from build123d import *

# Parameters (mm, degrees)
SKETCH1_W                  = 330
SKETCH1_H                  = 40
BOSS_EXTRUDE1_DEPTH        = 10
SKETCH2_W                  = 10.95
SKETCH2_H                  = 9
SKETCH2_W_2                = 8.1
SKETCH2_H_2                = 6.6
SKETCH2_H_3                = 6.8
SKETCH2_W_3                = 2.5
SKETCH2_H_4                = 4.6
CUT_EXTRUDE1_DEPTH         = 167.508258053
FILLET1_R                  = 2.5
LPATTERN1_COUNT            = 3
LPATTERN1_PITCH            = 70
FILLET1_OF_LPATTERN1_R     = 2.5
LPATTERN1_COL_COUNT        = 3
LPATTERN1_COL_PITCH        = 70
FILLET1_OF_LPATTERN1_COL_R = 2.5
SKETCH3_W                  = 10
SKETCH3_H                  = 9
CUT_EXTRUDE2_DEPTH         = 167.508258053
FILLET2_R                  = 20


with BuildPart() as part:
    # Sketch1 → Boss-Extrude1 (new body)
    with BuildSketch(Plane(origin=(0, 0, 0), x_dir=(1, 0, 0), z_dir=(0, 1, 0))):
        Rectangle(SKETCH1_W, SKETCH1_H)
    extrude(amount=BOSS_EXTRUDE1_DEPTH)

    # Sketch2 → Cut-Extrude1 (cut, through all)
    with BuildSketch(Plane(origin=(0, 10, 0), x_dir=(1, 0, 0), z_dir=(0, 1, 0))):
        with Locations((9.525, -15.5)):
            Rectangle(SKETCH2_W, SKETCH2_H)
        with Locations((0, -15.5)):
            Rectangle(SKETCH2_W_2, SKETCH2_H)
        with Locations((-9.525, -15.5)):
            Rectangle(SKETCH2_W, SKETCH2_H)
        with Locations((0, -7.7)):
            Rectangle(SKETCH2_W_2, SKETCH2_H_2)
        with Locations((0, -1)):
            Rectangle(SKETCH2_W_2, SKETCH2_H_3)
        with Locations((-5.3, -1)):
            Rectangle(SKETCH2_W_3, SKETCH2_H_3)
        with Locations((0, 4.7)):
            Rectangle(SKETCH2_W_2, SKETCH2_H_4)
        with Locations((5.3, -1)):
            Rectangle(SKETCH2_W_3, SKETCH2_H_3)
    cut_extrude1 = extrude(amount=-CUT_EXTRUDE1_DEPTH, mode=Mode.SUBTRACT)

    # Fillet1
    fillet1_edges = [part.edges().sort_by_distance(p)[0] for p in [
        (15, 5, 20),
        (-15, 5, 20),
    ]]
    fillet(fillet1_edges, radius=FILLET1_R)

    # LPattern1: Cut-Extrude1 ×3
    with Locations(*[(i * LPATTERN1_PITCH, 0, 0) for i in range(1, LPATTERN1_COUNT)]):
        add(cut_extrude1, mode=Mode.SUBTRACT)

    # Fillet1 of LPattern1
    fillet1_of_lpattern1_edges = [part.edges().sort_by_distance(p)[0] for p in [
        (85, 5, 20),
        (55, 5, 20),
        (155, 5, 20),
        (125, 5, 20),
    ]]
    fillet(fillet1_of_lpattern1_edges, radius=FILLET1_OF_LPATTERN1_R)

    # LPattern1 col: Cut-Extrude1 ×3
    with Locations(*[(-i * LPATTERN1_COL_PITCH, 0, 0) for i in range(1, LPATTERN1_COL_COUNT)]):
        add(cut_extrude1, mode=Mode.SUBTRACT)

    # Fillet1 of LPattern1 col
    fillet1_of_lpattern1_col_edges = [part.edges().sort_by_distance(p)[0] for p in [
        (-55, 5, 20),
        (-85, 5, 20),
        (-125, 5, 20),
        (-155, 5, 20),
    ]]
    fillet(fillet1_of_lpattern1_col_edges, radius=FILLET1_OF_LPATTERN1_COL_R)

    # Sketch3 → Cut-Extrude2 (cut, through all)
    with BuildSketch(Plane(origin=(0, 10, 0), x_dir=(1, 0, 0), z_dir=(0, 1, 0))):
        with Locations((-160, -15.5)):
            Rectangle(SKETCH3_W, SKETCH3_H)
    cut_extrude2 = extrude(amount=-CUT_EXTRUDE2_DEPTH, mode=Mode.SUBTRACT)

    # Mirror1: Cut-Extrude2 across plane
    add(cut_extrude2.mirror(Plane(origin=(0, 0, 0), x_dir=(0, 0, 1), z_dir=(1, 0, 0))), mode=Mode.SUBTRACT)

    # Fillet2
    fillet2_edges = [part.edges().sort_by_distance(p)[0] for p in [
        (-165, 5, -20),
        (165, 5, -20),
    ]]
    fillet(fillet2_edges, radius=FILLET2_R)


solid = part.part
Design review of the part built by this model. Coordinates are the model's own, in mm. A direction names the side the tool comes from. Coordinates: 2 decimals unless noted, no trailing zeros. Write each loop counter-clockwise with the first axis right and the second up, starting at its lowest first coordinate (ties: lowest second). Pieces come first, ordered by that corner, then holes. Notation, with made-up numbers: (-33.75, 81) - (-22.75, 81) arc R11 cw to (-22.75, 93) - close; hole circle Ø7 at (-6.5, -13.75). An arc over 180 degrees is marked (long way). Use one line per item in the form item = value.
Q1. Insertion check: pin 1 Ø6 at (x, y) = (-56.5, 6.5) entering from +Z; pin 2 Ø2 at (y, z) = (4, -0.5) entering from -X; pin 3 Ø3 at (x, y) = (-65, 5.5) entering from +Z; pin 4 Ø3.5 at (y, z) = (7, -4.5) entering from -X. Each pin has a flat end and moves straight along its axis. Give the tip position at first contact, or say it passes through.
Taken from the geometry:
pin_1 = 19.79
pin_2 = -165
pin_3 = 11
pin_4 = -164.81
Q2. Machinability: for faces 1 (the flat face through (146.55, 5, 1)), 2 (the flat face through (-154, 5, 11)), 3 (the flat face through (125, 5, 14)), 4 (the flat face through (-2, 0, -9)), 5 (the flat face through (74.05, 5, 8)), which of the approach directions +Z, -Z, +X, -X, +Y, -Y give a long, thin tool a straight path to every point of the face, cutting with its end or side? Answer none if there is none.
Taken from the geometry:
face_1 = +Y, -Y
face_2 = +Z, -X, +Y, -Y
face_3 = +Z, +X, +Y, -Y
face_4 = +Z, -Z, +X, -X, -Y
face_5 = +Z, +Y, -Y
Q3. For probe 1 along X at (y, z) = (2, 6); probe 2 along X at (y, z) = (6.25, 17.5); probe 3 along X at (y, z) = (7.75, -1), list the stretches that pass through material, from the lowest coordinate up.
Taken from the geometry:
probe_1 = -165 to -144.05, -135.95 to -74.05, -65.95 to -4.05, 4.05 to 65.95, 74.05 to 135.95, 144.05 to 165
probe_2 = -125 to -85, -55 to -15, 15 to 55, 85 to 125
probe_3 = -164.97 to -146.55, -133.45 to -76.55, -63.45 to -6.55, 6.55 to 63.45, 76.55 to 133.45, 146.55 to 164.97
Q4. Consider section A-A (x = 70). Write out the cut boundary in (y, z), plus the area to 3 significant figures.
Taken from the geometry:
outline = (0, -20) - (10, -20) - (10, -7) - (0, -7) - close
area = 130 mm^2
Q5. Consider section B-B (z = -13). Write out the cut boundary in (x, y).
Taken from the geometry:
outline = (-160.2, 0) - (160.2, 0) - (160.2, 10) - (-160.2, 10) - close
